Geometry: see drawing. Coordinates: mm, zero at the bounding-box minimum. Coordinates: 2 decimals unless noted, no trailing zeros. Loops run counter-clockwise (first coordinate to the right, second up) from the corner with the lowest first, then second, coordinate; pieces in that order, holes last. Notation, with made-up numbers: (-33, 76) -> (-8, 76) arc R32 cw to (-8, 112) -> close; hole circle Ø5 at (72, 64.25). An arc over 180 degrees is marked (long way). Put each result on its own line as item: value. Start each with the question number.
1) Contact query for a flat-ended pin moving along its axis: P1, Ø1, axis at x = 150, z = 2.5, coming from the -Y side. Output: stop coordinate, or through.
2) Cut plane D-D (x = 141). Return the cut outline in (y, z), plus the area to 3 significant figures.
3) Cut plane C-C (y = 23.5). Return the cut outline in (x, z).
4) Cut plane A-A (x = 82.5). Return the cut outline in (y, z), plus the area to 3 significant figures.
5) Material intervals for L1, parallel to Y at x = 75, z = 3.25; L2, parallel to Y at x = 19.5, z = 2.5; L3, parallel to Y at x = 100, z = 1, sorted ascending.
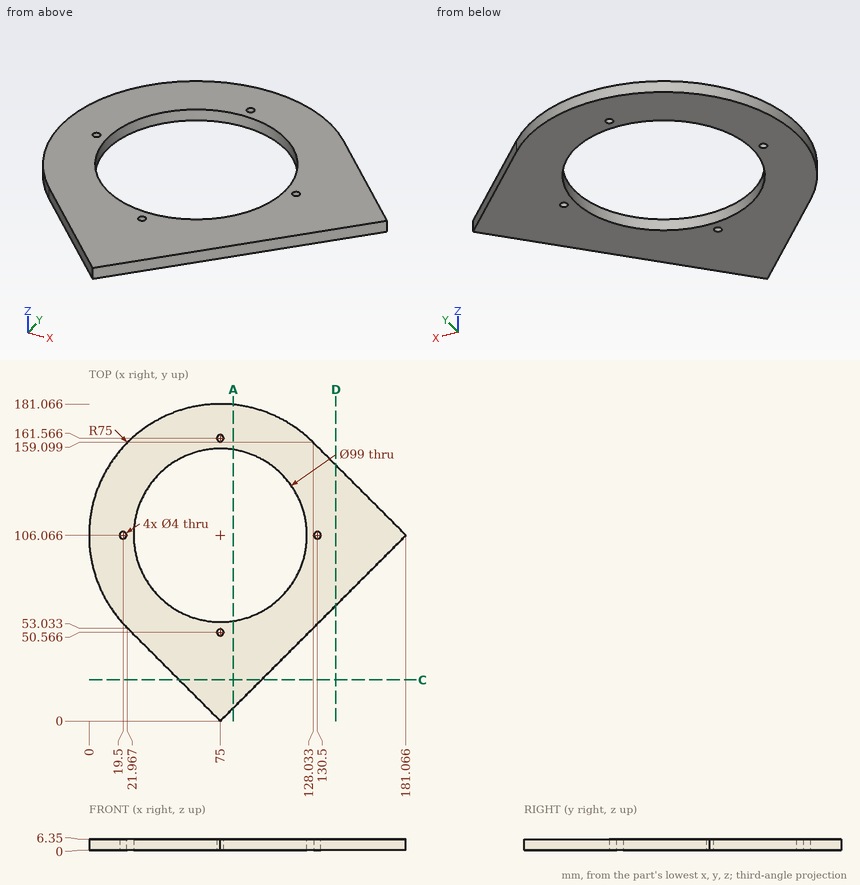
Results found:
1. P1: stops at y = 74.5
2. outline: (66, 0) -> (146.13, 0) -> (146.13, 6.35) -> (66, 6.35) -> close
2. area: 509 mm2
3. outline: (51.5, 0) -> (98.5, 0) -> (98.5, 6.35) -> (51.5, 6.35) -> close
4. outline: (7.5, 0) -> (57.14, 0) -> (57.14, 6.35) -> (7.5, 6.35) -> close; (154.99, 0) -> (180.69, 0) -> (180.69, 6.35) -> (154.99, 6.35) -> close
4. area: 478 mm2
5. L1: y = 0 to 48.57, 52.57 to 56.57, 155.57 to 159.57, 163.57 to 181.07
5. L2: y = 55.62 to 104.07, 108.07 to 156.51
5. L3: y = 25 to 63.34, 148.79 to 176.78
